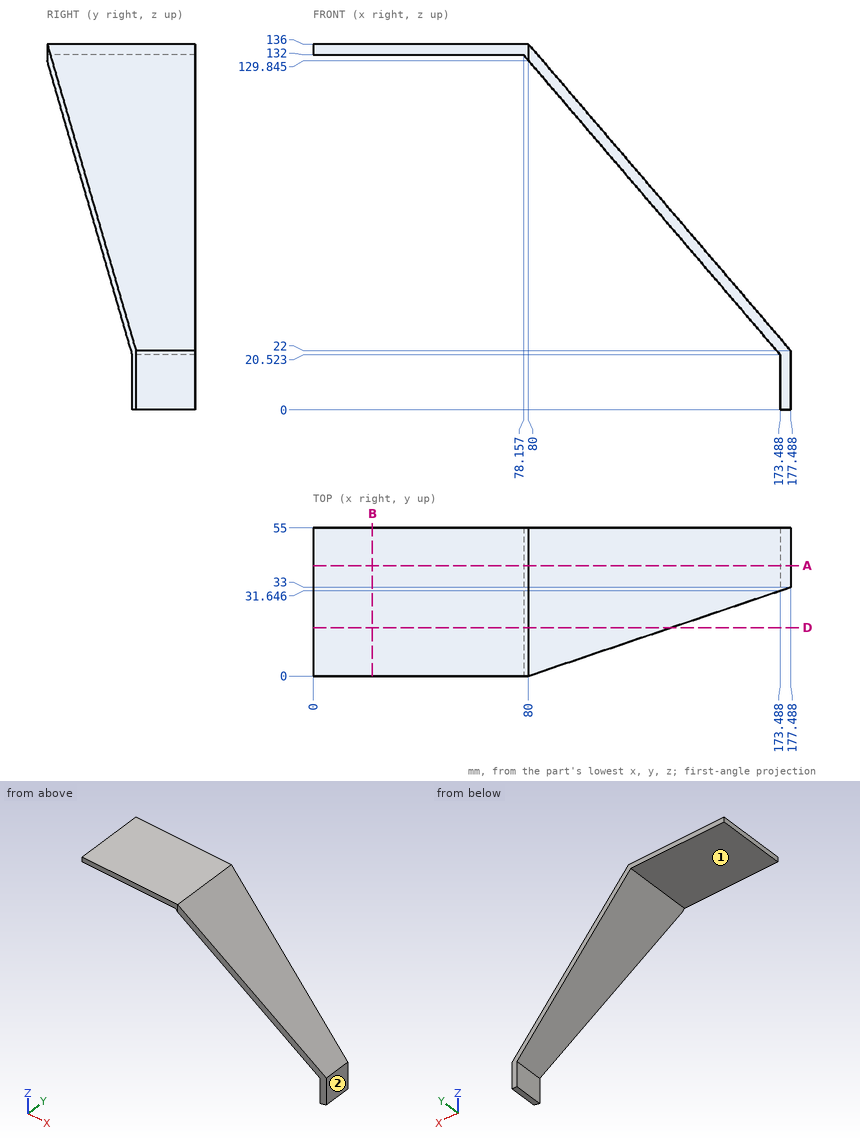
Here's the drawing with two shaded views (mm, measured from the low corner). I have some questions. A direction names the side the tool comes from. Coordinates: 2 decimals unless noted, no trailing zeros. Order: outer loops, then holes, each group sorted by start corner. A loop starts at its lowest first (then second) coordinate and runs counter-clockwise, first axis right, second up. Notation, with made-up numbers: (53, 54.25) - (90, 54.25) arc R15 cw to (90, 64.25) - close; hole circle Ø5 at (57.5, -38). An arc over 180 degrees is marked (long way). Answer in a Markdown table with one row per item. Add a question column.
(1) If we section it at A-A, the plane y = 41: Please give me the cut outline in (x, z).
(2) If we section it at D-D, the plane y = 18: Please give me the cut outline in (x, z) (1 decimal).
(3) If we section it at B-B, the plane x = 22: Please give me the cut outline in (y, z).
(4) On a 3-axis mill with a long thin cutter (end or side, diameter ignored), from which of +Z, -Z, +X, -X, +Y, -Y can I reach the whole of each face in a straight line? I mean the marked faces 1 and 2. Say none if no direction works.
(5) Will these pins go through, and if not, where does the flat tip stop? pin 1 (16.5 mm diameter, centred on x = 37.5, y = 19, fed in from -Z); pin 2 (1 mm diameter, centred on y = 29, z = 102, fed in from +X); pin 3 (6 mm diameter, centred on x = 106, y = 25.5, fed in from -Z) (1 decimal).
(6) I need wall thicknesses on L1, parallel to Z at x = 68.5, y = 4; L2, parallel to X at y = 35.5, z = 116 (1 decimal); L3, parallel to X at y = 20, z = 72.5 (1 decimal). Which ranges of each line are inside material? Lowest first, please.
Results are:
| question | item | result |
|---|---|---|
| 1 | outline | (0, 132) - (78.16, 132) - (173.49, 20.52) - (173.49, 0) - (177.49, 0) - (177.49, 22) - (80, 136) - (0, 136) - close |
| 2 | outline | (0, 132) - (78.2, 132) - (133.2, 67.7) - (133.2, 73.8) - (80, 136) - (0, 136) - close |
| 3 | outline | (0, 132) - (55, 132) - (55, 136) - (0, 136) - close |
| 4 | face 1 | -Z, -X, +Y, -Y |
| 4 | face 2 | +Z, -Z, +X, +Y, -Y |
| 5 | pin 1 | stops at z = 132 |
| 5 | pin 2 | stops at x = 109.5 |
| 5 | pin 3 | stops at z = 95.9 |
| 6 | L1 | z = 132 to 136 |
| 6 | L2 | x = 91.8 to 97.1 |
| 6 | L3 | x = 129 to 134.3 |
